```python
from build123d import *

# Parameters (mm, degrees)
F0_R     = 3.5
F0_R_2   = 10.5
F1_DEPTH = 6
F2_R     = 10.5
F2_R_2   = 6
F3_DEPTH = 16
F4_R     = 17
F4_R_2   = 10.5
F5_DEPTH = 6
F6_R     = 5
F7_R     = 1
F8_SIZE  = 0.2
F9_SIZE  = 0.2


with BuildPart() as f1:
    # F0 (on Front) → F1 (new body)
    with BuildSketch(Plane.XZ):
        with BuildLine():
            Line((-31.5, 6), (-31.5, -6))
            Line((-31.5, -6), (-17, -8.485281))
            ThreePointArc((-17, -8.485281), (-19, 0), (-17, 8.485281))
            Line((-17, 8.485281), (-31.5, 6))
        make_face()
        with Locations((-24, 0)):
            Circle(F0_R, mode=Mode.SUBTRACT)
        with BuildLine():
            ThreePointArc((-17, 8.485281), (-19, 0), (-17, -8.485281))
            ThreePointArc((-17, -8.485281), (0, -19), (17, -8.485281))
            ThreePointArc((17, -8.485281), (18.493242, -4.358899), (19, 0))
            ThreePointArc((19, 0), (18.493242, 4.358899), (17, 8.485281))
            ThreePointArc((17, 8.485281), (0, 19), (-17, 8.485281))
        make_face()
        Circle(F0_R_2, mode=Mode.SUBTRACT)
        with BuildLine():
            ThreePointArc((19, 0), (18.493242, -4.358899), (17, -8.485281))
            Line((17, -8.485281), (31.5, -6))
            Line((31.5, -6), (31.5, 6))
            Line((31.5, 6), (17, 8.485281))
            ThreePointArc((17, 8.485281), (18.493242, 4.358899), (19, 0))
        make_face()
        with Locations((24, 0)):
            Circle(F0_R, mode=Mode.SUBTRACT)
    extrude(amount=F1_DEPTH)

    # F2 (on Front) → F3 (join)
    with BuildSketch(Plane.XZ):
        Circle(F2_R)
        Circle(F2_R_2, mode=Mode.SUBTRACT)
    extrude(amount=F3_DEPTH)

    # F4 (on face) → F5 (join)
    with BuildSketch(Plane.XZ.offset(6)):
        Circle(F4_R)
        Circle(F4_R_2, mode=Mode.SUBTRACT)
    extrude(amount=F5_DEPTH)

    # F6
    f6_edges = [f1.edges().sort_by_distance(p)[0] for p in [
        (-17, -3, -8.485281),
        (17, -3, -8.485281),
        (17, -3, 8.485281),
        (-17, -3, 8.485281),
    ]]
    fillet(f6_edges, radius=F6_R)

    # F7
    f7_edges = [f1.edges().sort_by_distance(p)[0] for p in [
        (-31.5, -3, -6),
        (31.5, -3, -6),
        (31.5, -3, 6),
        (-31.5, -3, 6),
    ]]
    fillet(f7_edges, radius=F7_R)

    # F8
    f8_edges = [f1.edges().sort_by_distance(p)[0] for p in [
        (-17, -12, 0),
        (24.994126, -6, -7.115098),
        (31.264505, -6, -5.801434),
        (17.408545, -6, -8.843659),
        (31.5, -6, 0),
        (0, -6, -19),
        (31.264505, -6, 5.801434),
        (-17.408545, -6, -8.843659),
        (24.994126, -6, 7.115098),
        (-24.994126, -6, -7.115098),
        (17.408545, -6, 8.843659),
        (-31.264505, -6, -5.801434),
        (0, -6, 19),
        (-31.5, -6, 0),
        (-17.408545, -6, 8.843659),
        (-31.264505, -6, 5.801434),
        (-24.994126, -6, 7.115098),
        (-27.5, -6, 0),
        (-17, -6, 0),
        (20.5, -6, 0),
        (24.994126, 0, 7.115098),
        (31.264505, 0, 5.801434),
        (17.408545, 0, 8.843659),
        (31.5, 0, 0),
        (0, 0, 19),
        (31.264505, 0, -5.801434),
        (-17.408545, 0, 8.843659),
        (24.994126, 0, -7.115098),
        (-24.994126, 0, 7.115098),
        (17.408545, 0, -8.843659),
        (-31.264505, 0, 5.801434),
        (0, 0, -19),
        (-31.5, 0, 0),
        (-17.408545, 0, -8.843659),
        (-31.264505, 0, -5.801434),
        (-24.994126, 0, -7.115098),
        (-27.5, 0, 0),
        (20.5, 0, 0),
        (-6, 0, 0),
    ]]
    chamfer(f8_edges, length=F8_SIZE)

    # F9
    f9_edges = [f1.edges().sort_by_distance(p)[0] for p in [
        (-10.5, -16, 0),
        (-6, -16, 0),
    ]]
    chamfer(f9_edges, length=F9_SIZE)


solid = f1.part
```
Verification items for the finished model (mm, model axes). A direction names the side the tool comes from. Round coordinates to 2 decimals unless told otherwise and drop trailing zeros. Write each loop counter-clockwise with the first axis right and the second up, starting at its lowest first coordinate (ties: lowest second). Pieces come first, ordered by that corner, then holes. Notation, with made-up numbers: (-15, -29.75) -> (-11, -29.75) arc R22 ccw to (-11, -12.75) -> close; hole circle Ø10 at (51, 11). An arc over 180 degrees is marked (long way). Write each question's results on one line, items separated by ' | '. Start each with the question number.
1. Material ranges on probe 1 along Y at (x, z) = (2.5, -14.5); probe 2 along X at (y, z) = (-8, 4.5); probe 3 along Y at (x, z) = (20.5, -6), recorded low to high. Write a range as from..to.
2. Cross-section at A-A (y = -9). Enter the section's corners in (x, z), then the cut area to 3 significant figures.
3. Depth check by flat-ended pin: P1, Ø2, axis at x = -11.5, y = -4.5, coming from the +Z side; P2, Ø11, axis at x = -24, z = 0, coming from the -Y side; P3, Ø2, axis at x = -6, y = -6, coming from the -Z side. Enter the tip coordinate at first touch or a pass-through.
4. Set-up check for faces 1 (the cylindrical face through (0, -3, -19)), 2 (the cylindrical face through (9.139, -8.961, 14.334)): record each of +Z, -Z, +X, -X, +Y, -Y from which the full face is reachable in a straight line by a thin tool's end or side.
5. Cross-section at C-C (z = -1.5). Count the separate pieces of the cut face and the enclosed holes in it, then the cut area to 3 significant figures.
6. Cross-section at D-D (y = -14.25). Enter the section's corners in (x, z), then the cut area to 3 significant figures.
7. Cross-section at B-B (x = -24). Enter the section's corners in (y, z), then the cut area to 3 significant figures.
Solutions:
1) probe 1: y = -12..0 | probe 2: x = -16.39..-3.97, 3.97..16.39 | probe 3: y = -6..0
2) outline: circle Ø34 at (0, 0); hole circle Ø12 at (0, 0) | area: 795 mm2
3) P1: stops at z = 15.84 | P2: stops at y = -6 | P3: stops at z = -18.32
4) face 1: -Z, +Y, -Y | face 2: -Y
5) separate pieces: 4 | enclosed holes: 0 | area: 402 mm2
6) outline: circle Ø21 at (0, 0); hole circle Ø12 at (0, 0) | area: 233 mm2
7) outline: (-6, -7.08) -> (-5.8, -7.29) -> (-0.2, -7.29) -> (0, -7.08) -> (0, -3.7) -> (-0.2, -3.5) -> (-5.8, -3.5) -> (-6, -3.7) -> close; (-6, 3.7) -> (-5.8, 3.5) -> (-0.2, 3.5) -> (0, 3.7) -> (0, 7.08) -> (-0.2, 7.29) -> (-5.8, 7.29) -> (-6, 7.08) -> close | area: 45.3 mm2
